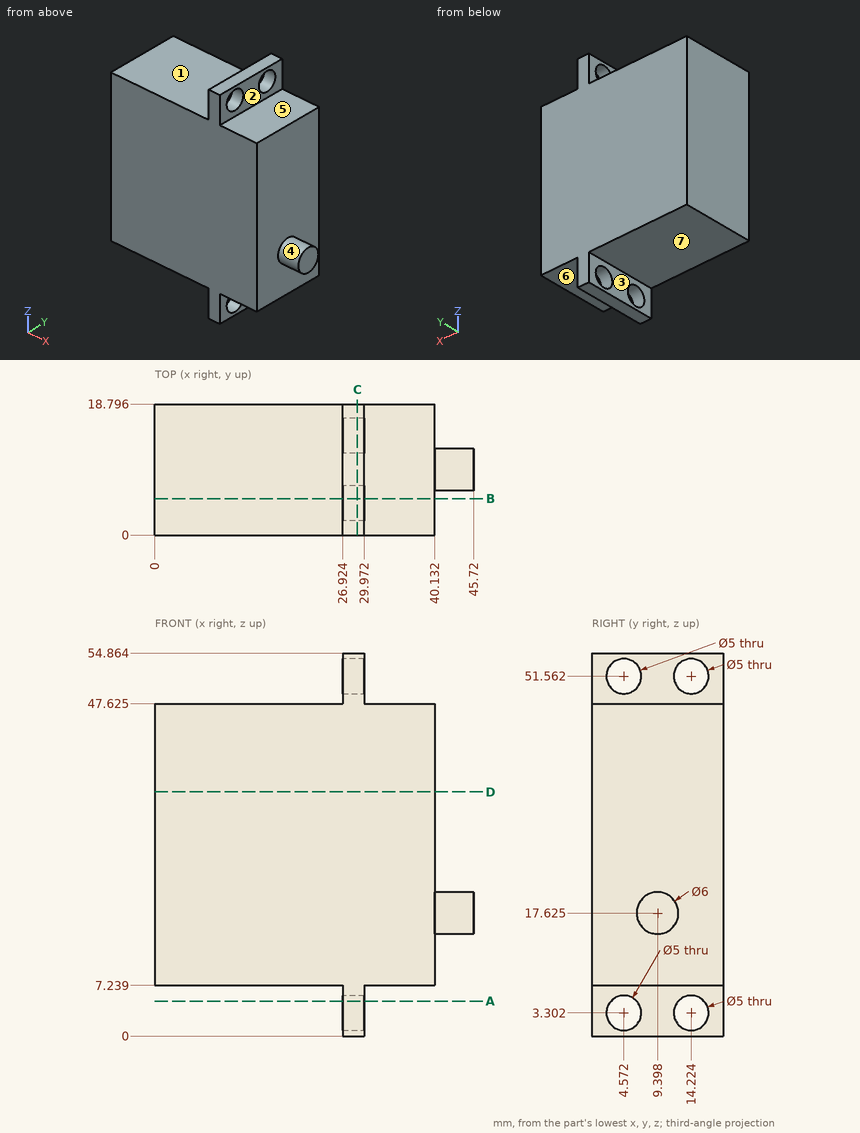
Check sheet for the drawn part. Datum: minimum x, y, z corner. Units: mm. A direction names the side the tool comes from. Round coordinates to 2 decimals unless told otherwise and drop trailing zeros. Order: outer loops, then holes, each group sorted by start corner. A loop starts at its lowest first (then second) coordinate and runs counter-clockwise, first axis right, second up.
1. Release check for a two-part mould opening along X. For the marked faces 1, 2 and 3 record: +X half, -X half, draft (parallel to the pull), parting line (faces both ways), or undercut.
Final values:
face 1: draft
face 2: +X half
face 3: -X half
2. Access from +Z, -Z, +X, -X, +Y, -Y to the whole of each face (thin tool, end or side, straight path). Record for the marked faces 4, 5, 6 and 7.
Final values:
face 4: +X
face 5: +Z, +X, +Y, -Y
face 6: -Z, +X, +Y, -Y
face 7: -Z, -X, +Y, -Y
3. Go/stop test with flat-tipped pins: P1, Ø5, axis at x = 33.5, y = 14, coming from the -Z side; P2, Ø1.5, axis at x = 31, y = 5.5, coming from the +Z side (3 decimals); P3, Ø2, axis at y = 4.5, z = 28, coming from the +X side; P4, Ø3, axis at y = 4.572, z = 3.302, coming from the -X side. Record where each tip stops, or that it passes through.
Final values:
P1: stops at z = 7.24
P2: stops at z = 47.625
P3: stops at x = 40.13
P4: passes through
4. Section check B-B on y = 5.25. Record the cut outline in (x, z) (3 decimals), then the cut area to 3 significant figures.
Final values:
outline: (0, 7.239) - (26.924, 7.239) - (26.924, 5.708) - (29.972, 5.708) - (29.972, 7.239) - (40.132, 7.239) - (40.132, 47.625) - (29.972, 47.625) - (29.972, 49.156) - (26.924, 49.156) - (26.924, 47.625) - (0, 47.625) - close; (26.924, 0) - (29.972, 0) - (29.972, 0.896) - (26.924, 0.896) - close; (26.924, 53.968) - (29.972, 53.968) - (29.972, 54.864) - (26.924, 54.864) - close
area: 1,640 mm2
5. Section check A-A on z = 5. Record the cut outline in (x, y), then the cut area to 3 significant figures.
Final values:
outline: (26.92, 0) - (29.97, 0) - (29.97, 2.74) - (26.92, 2.74) - close; (26.92, 6.41) - (29.97, 6.41) - (29.97, 12.39) - (26.92, 12.39) - close; (26.92, 16.06) - (29.97, 16.06) - (29.97, 18.8) - (26.92, 18.8) - close
area: 34.9 mm2
6. Thickness scan on L1, parallel to X at y = 15.75, z = 34; L2, parallel to Z at x = 6, y = 9.5 (3 decimals); L3, parallel to Z at x = 28, y = 3.75. Record the ranges inside material, lowest first.
Final values:
L1: x = 0 to 40.13
L2: z = 7.239 to 47.625
L3: z = 0 to 0.94, 5.66 to 49.2, 53.92 to 54.86
7. Section check D-D on z = 35. Record the cut outline in (x, y).
Final values:
outline: (0, 0) - (40.13, 0) - (40.13, 18.8) - (0, 18.8) - close
8. Section check C-C on x = 29. Record the cut outline in (y, z), then the cut area to 3 significant figures.
Final values:
outline: (0, 0) - (18.8, 0) - (18.8, 54.86) - (0, 54.86) - close; hole circle Ø5 at (4.57, 3.3); hole circle Ø5 at (4.57, 51.56); hole circle Ø5 at (14.22, 3.3); hole circle Ø5 at (14.22, 51.56)
area: 953 mm2
